The listing builds one solid part. Answer for the finished solid, in the listing's coordinates (mm). Face numbers are marked on the shaded views. A direction names the side the tool comes from. Round coordinates to 2 decimals unless told otherwise and drop trailing zeros. Write each loop counter-clockwise with the first axis right and the second up, starting at its lowest first coordinate (ties: lowest second). Pieces come first, ordered by that corner, then holes.
from build123d import *

# Parameters (mm, degrees)
F1_DEPTH = 10


with BuildPart() as f1:
    # F0 (on Front) → F1 (new body)
    with BuildSketch(Plane.XZ):
        with BuildLine():
            ThreePointArc((39.68627, -5), (39.92149, -2.504917), (40, 0))
            ThreePointArc((40, 0), (39.92149, 2.504917), (39.68627, 5))
            ThreePointArc((39.68627, 5), (28.284271, 28.284271), (5, 39.68627))
            ThreePointArc((5, 39.68627), (0, 40), (-5, 39.68627))
            ThreePointArc((-5, 39.68627), (-28.284271, 28.284271), (-39.68627, 5))
            ThreePointArc((-39.68627, 5), (-40, 0), (-39.68627, -5))
            ThreePointArc((-39.68627, -5), (-28.284271, -28.284271), (-5, -39.68627))
            ThreePointArc((-5, -39.68627), (0, -40), (5, -39.68627))
            ThreePointArc((5, -39.68627), (28.284271, -28.284271), (39.68627, -5))
        make_face()
        with BuildLine():
            ThreePointArc((-5, -30.594117), (-21.92031, -21.92031), (-30.594117, -5))
            Line((-30.594117, -5), (-5, -5))
            Line((-5, -5), (-5, -30.594117))
        make_face(mode=Mode.SUBTRACT)
        with BuildLine():
            Line((5, -30.594117), (5, -5))
            Line((5, -5), (30.594117, -5))
            ThreePointArc((30.594117, -5), (21.92031, -21.92031), (5, -30.594117))
        make_face(mode=Mode.SUBTRACT)
        with BuildLine():
            ThreePointArc((-30.594117, 5), (-21.92031, 21.92031), (-5, 30.594117))
            Line((-5, 30.594117), (-5, 5))
            Line((-5, 5), (-30.594117, 5))
        make_face(mode=Mode.SUBTRACT)
        with BuildLine():
            ThreePointArc((0, 2.5), (1.767767, 1.767767), (2.5, 0))
            ThreePointArc((2.5, 0), (1.767767, -1.767767), (0, -2.5))
            ThreePointArc((0, -2.5), (-1.767767, -1.767767), (-2.5, 0))
            ThreePointArc((-2.5, 0), (-1.767767, 1.767767), (0, 2.5))
        make_face(mode=Mode.SUBTRACT)
        with BuildLine():
            Line((30.594117, 5), (5, 5))
            Line((5, 5), (5, 30.594117))
            ThreePointArc((5, 30.594117), (21.92031, 21.92031), (30.594117, 5))
        make_face(mode=Mode.SUBTRACT)
    extrude(amount=F1_DEPTH)


solid = f1.part
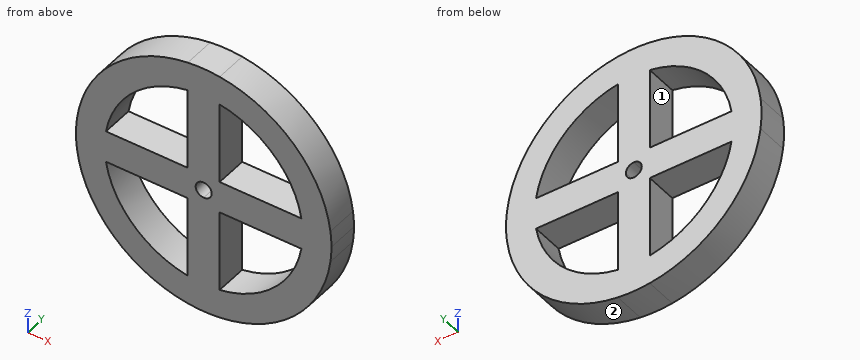
1. A tool of negligible diameter and unlimited length cuts with its end or side. For the marked faces 1 and 2, from which of +Z, -Z, +X, -X, +Y, -Y can it reach the whole face along a straight path? Write none if from no direction.
Geometry says:
face 1: +Y, -Y
face 2: -Z, +X, +Y, -Y
2. Straight lines are drawn through the part: line 1 along Z through (x, y) = (22.5, -8.75); line 2 along Z through (x, y) = (25.5, -2); line 3 along X through (y, z) = (-3.5, -12.5). For each, find the intervals that lie inside material, in ascending order.
Geometry says:
line 1: z = -33.07 to -21.32, -5 to 5, 21.32 to 33.07
line 2: z = -30.82 to -17.63, -5 to 5, 17.63 to 30.82
line 3: x = -38 to -28.37, -5 to 5, 28.37 to 38
3. Section A-A on y = -7 is taken. Determine the outline of the cut face in (x, z).
Geometry says:
outline: (-39.69, -5) arc R40 ccw to (-5, -39.69) arc R40 ccw to (5, -39.69) arc R40 ccw to (39.69, -5) arc R40 ccw to (40, 0) arc R40 ccw to (39.69, 5) arc R40 ccw to (5, 39.69) arc R40 ccw to (-5, 39.69) arc R40 ccw to (-39.69, 5) arc R40 ccw to start; hole (-30.59, -5) arc R31 ccw to (-5, -30.59) - (-5, -5) - close; hole (-30.59, 5) - (-5, 5) - (-5, 30.59) arc R31 ccw to start; hole circle Ø5 at (0, 0); hole (5, -30.59) arc R31 ccw to (30.59, -5) - (5, -5) - close; hole (5, 5) - (30.59, 5) arc R31 ccw to (5, 30.59) - close
4. Section D-D on x = -1 is taken. Determine the outline of the cut face in (y, z).
Geometry says:
outline: (-10, -39.99) - (0, -39.99) - (0, -2.29) - (-10, -2.29) - close; (-10, 2.29) - (0, 2.29) - (0, 39.99) - (-10, 39.99) - close
5. Section B-B on z = 28 is taken. Determine the outline of the cut face in (x, y).
Geometry says:
outline: (-28.57, -10) - (-13.3, -10) - (-13.3, 0) - (-28.57, 0) - close; (-5, -10) - (5, -10) - (5, 0) - (-5, 0) - close; (13.3, -10) - (28.57, -10) - (28.57, 0) - (13.3, 0) - close
6. Section C-C on x = 24 is taken. Determine the outline of the cut face in (y, z).
Geometry says:
outline: (-10, -32) - (0, -32) - (0, -19.62) - (-10, -19.62) - close; (-10, -5) - (0, -5) - (0, 5) - (-10, 5) - close; (-10, 19.62) - (0, 19.62) - (0, 32) - (-10, 32) - close
7. Given pin 1 (1.5 mm diameter, centred on y = -4.5, z = -16, fed in from +X); pin 2 (4 mm diameter, centred on y = -5.5, z = -23, fed in from +X); pin 3 (5 mm diameter, centred on x = -17, y = -4.5, fed in from -Z); pin 4 (10 mm diameter, centred on x = 19, z = 18.5, fed in from +Y), each flat-ended and moving along its own axis, determine where each tip first touches the part or whether it passes through.
Geometry says:
pin 1: stops at x = 36.98
pin 2: stops at x = 34.04
pin 3: stops at z = -37.28
pin 4: stops at y = 0
